Could you check a few things on this model? Use its own coordinates, in mm. A direction names the side the tool comes from. Give positions to 0.01 mm unless a question says otherwise; leave off trailing zeros. Order: outer loops, then holes, each group sorted by start corner. A loop starts at its lowest first (then second) coordinate and runs counter-clockwise, first axis right, second up. Notation, with made-up numbers: M 1,-39.5 L 24,-39.5 A23 cw 24,-8.5 Z; hole C 46.25,-0.75 d6. An arc over 180 degrees is marked long. Answer in a Markdown table with one row per item. Add a question column.
Autodesk Inventor part; units mm, degrees
ref_plane "YZ Plane" through (0, 0, 0) normal (1, 0, 0) x (0, 1, 0)
ref_plane "XZ Plane" through (0, 0, 0) normal (0, 1, 0) x (-1, 0, 0)
ref_plane "XY Plane" through (0, 0, 0) normal (0, 0, 1) x (1, 0, 0)
sketch "スケッチ1" plane through (0, 0, 0) normal (0, 1, 0) x (-1, 0, 0)
  circle A0 centre (15, 44.75) radius 2
  circle A1 centre (5, 44.75) radius 2
  circle A2 centre (10, 30) radius 3
  circle A3 centre (15, -4.75) radius 2
  circle A4 centre (5, -4.75) radius 2
  circle A5 centre (10, 30) radius 3
  line L0 (0, 0) -> (0, 40)
  line L1 (20, 0) -> (0, 0)
  line L2 (20, 40) -> (20, 0)
  line L3 (0, 40) -> (20, 40)
  line L4 (0, 40) -> (20, 40)
  line L5 (20, 45.25) -> (20, 40)
  arc A6 (20, 45.25) -> (18, 47.447) centre (18.0097, 45.4471) ccw
  line L6 (2, 47.447) -> (18, 47.447)
  arc A7 (2, 47.447) -> (0, 45.25) centre (1.9903, 45.4471) ccw
  line L7 (0, 40) -> (0, 45.25)
  circle A8 centre (15, 44.75) radius 2
  circle A9 centre (5, 44.75) radius 2
  line L8 (20, 0) -> (0, 0)
  line L9 (0, -5.25) -> (0, 0)
  arc A10 (0, -5.25) -> (2, -7.25) centre (2, -5.25) ccw
  line L10 (18, -7.25) -> (2, -7.25)
  arc A11 (18, -7.25) -> (20, -5.25) centre (18, -5.25) ccw
  line L11 (20, 0) -> (20, -5.25)
  circle A12 centre (5, -4.75) radius 2
  circle A13 centre (15, -4.75) radius 2
  line L12 (-8, 50.197) -> (28, 50.197)
  line L13 (30, 48.197) -> (30, -7.803)
  line L14 (28, -9.803) -> (-8, -9.803)
  line L15 (-10, -7.803) -> (-10, 48.197)
  arc A14 (30, 48.197) -> (28, 50.197) centre (28, 48.197) ccw
  arc A15 (-8, 50.197) -> (-10, 48.197) centre (-8, 48.197) ccw
  arc A16 (-10, -7.803) -> (-8, -9.803) centre (-8, -7.803) ccw
  arc A17 (28, -9.803) -> (30, -7.803) centre (28, -7.803) ccw
  line L16 (45.2724, 20.197) -> (-29.952, 20.197)
  line L17 (25, 53.3822) -> (25, -21.2286)
  line L18 (-5, 50.197) -> (-5, -9.803)
  line L19 (6.5, 45) -> (13.5, 45)
  line L20 (13.5, 45) -> (13.5, 40)
  line L21 (6.5, 40) -> (6.5, 45)
  line L22 (0, 40) -> (20, 40)
  point P0 (0, -4.75)
  point P1 (-10, 50.197)
  point P2 (30, -9.803)
  point P3 (30, 50.197)
  point P4 (10, 47.447)
  point P5 (10, 50.197)
  point P6 (-5, 20.197)
  point P7 (-5, 20.197)
  point P8 (25, 20.197)
  point P9 (25, 50.197)
  point P10 (25, -9.803)
  dimension "d0" = 40
  dimension "d1" = 60
  dimension "d2" = 2.75
  dimension "d3" = 10
  dimension "d4" = 2
  dimension "d5" = 30
  dimension "d6" = 5
  dimension "d7" = 5
  dimension "d8" = 60
  dimension "d9" = 0
  dimension "d22" = 2.75
  dimension "d23" = 2
  dimension "d24" = 2
  dimension "d25" = 10
  dimension "d26" = 15
  dimension "d27" = 5.447
  dimension "d28" = 10
  dimension "d29" = 20
  dimension "d30" = 20.197
extrude "押し出し1" add sketch "スケッチ1" along normal blind 5 contours A0 L20 L19 | A0 L19 A1 L21 L3 L7 A7 L6 A6 L5 L20 | L19 L21 A1 | L5 A6 L6 A7 L7 L0 L16 L18 L12 L17 L2 | L16 L17 L14 L18 L0 L9 A10 L10 A11 L11 L2 | L11 A11 L10 A10 L9 L1 | L17 L12 A14 L13 L16 | L16 L13 A17 L14 L17 | L18 L14 A16 L15 L16 | L16 L15 A15 L12 L18 | A3 | A4 picked at (15.8139, 44.6736) picked at (4.1802, 44.7383)
hole "穴1" at (5, 0, 20.197) at (-25, 0, 20.197) direction (0, 1, 0) diameter 4 end through all
sketch "スケッチ2" plane through (0, 5, 0) normal (0, 1, 0) x (1, 0, 0)
  circle A0 centre (5, -20.197) radius 2
  circle A1 centre (-25, -20.197) radius 2
  line L0 (-28, -50.197) -> (8, -50.197)
  arc A2 (8, -50.197) -> (10, -48.197) centre (8, -48.197) ccw
  line L1 (10, -48.197) -> (10, 7.803)
  arc A3 (10, 7.803) -> (8, 9.803) centre (8, 7.803) ccw
  line L2 (8, 9.803) -> (-28, 9.803)
  arc A4 (-28, 9.803) -> (-30, 7.803) centre (-28, 7.803) ccw
  line L3 (-30, 7.803) -> (-30, -48.197)
  arc A5 (-30, -48.197) -> (-28, -50.197) centre (-28, -48.197) ccw
  line L4 (-20, -40) -> (-20, 0)
  line L5 (-20, 0) -> (0, 0)
  line L6 (0, 0) -> (0, -40)
  line L7 (0, -40) -> (-6.5, -40)
  line L8 (-6.5, -40) -> (-6.5, -45)
  line L9 (-6.5, -45) -> (-13.5, -45)
  line L10 (-13.5, -45) -> (-13.5, -40)
  line L11 (-13.5, -40) -> (-20, -40)
  line L12 (-6, -40.5) -> (0.5, -40.5)
  line L13 (0.5, -40.5) -> (0.5, 0.5)
  line L14 (0.5, 0.5) -> (-20.5, 0.5)
  line L15 (-20.5, 0.5) -> (-20.5, -40.5)
  line L16 (-20.5, -40.5) -> (-14, -40.5)
  line L17 (-14, -40.5) -> (-14, -45.5)
  line L18 (-14, -45.5) -> (-6, -45.5)
  line L19 (-6, -45.5) -> (-6, -40.5)
  dimension "d19" = 0.5
extrude "押し出し2" cut sketch "スケッチ2" against normal blind 10 contours L19 L18 L17 L16 L15 L14 L13 L12
sketch "スケッチ3" plane through (0, 5, 0) normal (0, 1, 0) x (1, 0, 0)
  line L0 (10, -48.197) -> (10, 7.803)
  arc A0 (8, -50.197) -> (10, -48.197) centre (8, -48.197) ccw
  line L1 (-28, -50.197) -> (8, -50.197)
  arc A1 (-30, -48.197) -> (-28, -50.197) centre (-28, -48.197) ccw
  line L2 (-30, 7.803) -> (-30, -48.197)
  arc A2 (-28, 9.803) -> (-30, 7.803) centre (-28, 7.803) ccw
  line L3 (8, 9.803) -> (-28, 9.803)
  arc A3 (10, 7.803) -> (8, 9.803) centre (8, 7.803) ccw
  line L4 (6.2, -46.397) -> (6.2, 6.003)
  line L5 (6.2, 6.003) -> (-26.2, 6.003)
  line L6 (-26.2, 6.003) -> (-26.2, -46.397)
  line L7 (-26.2, -46.397) -> (6.2, -46.397)
  point P0 (0, 0)
  dimension "d31" = 3.8
extrude "押し出し3" cut sketch "スケッチ3" against normal blind 3
equation "\"d5\" = 0.5 * d1"
equation "\"d6\" = 0.5 * d3"
equation "\"d8\" = d1"
properties part number "servo_cover2_3D プリント"
1. Suppose I cut it at A-A on y = 1.05. List the corners of the cut face in (x, z) for me.
2. Suppose I cut it at B-B on x = -25. List the corners of the cut face in (y, z) for me.
3. Thinking about a two-plate mould opening in X: for faces 1 (the flat face through (7.5, 2, 19.8)), 2 (the flat face through (-26.2, 4, 34)), 3 (the flat face through (-10, 3, 45.5)), 4 (the cylindrical face through (9.43, 0.986, 49.596)), which applies, pulls with the +X half, pulls with the -X half, needs draft (parallel to the pull), parting line crosses it, or undercut?
4. Suppose I cut it at C-C on z = 6. List the corners of the cut face in (x, y) for me, plus the area to 3 significant figures.
5. Suppose I cut it at D-D on y = 4.3. List the corners of the cut face in (x, z) for me.
6. If I drill on line 1 along Z through (x, y) = (-13.5, 0.85); line 2 along Z through (x, y) = (-4, 4.25); line 3 along X through (y, z) = (1.15, 1), over which ranges is the centre line in solid material (lowest first)? Write a range as [from, to].
7. Will these pins go through, and if not, where does the flat tip stop? P1, Ø1.5, axis at y = 3.5, z = 42, coming from the +X side; P2, Ø1.5, axis at x = -6.5, y = 3, coming from the +Z side; P3, Ø0.9, axis at y = 3, z = 38, coming from the -X side; P4, Ø3, axis at x = -25, z = 20.197, coming from the +Y side.
8. For faces 5 (the flat face through (6.2, 4, 6)), 6 (the flat face through (-14, 3, 43)), 7 (the flat face through (-10, 4, 46.397)), 8 (the flat face through (-26.2, 4, 6)), which set-ups out of +Z, -Z, +X, -X, +Y, -Y let a thin tool reach every point of the face, with its end or its side?
Findings below:
| question | item | result |
|---|---|---|
| 1 | outline | M -30,-7.8 A2 ccw -28,-9.8 L 8,-9.8 A2 ccw 10,-7.8 L 10,48.2 A2 ccw 8,50.2 L -28,50.2 A2 ccw -30,48.2 Z; hole C -25,20.2 d4; hole M -20.5,-0.5 L 0.5,-0.5 L 0.5,40.5 L -6,40.5 L -6,45.5 L -14,45.5 L -14,40.5 L -20.5,40.5 Z; hole C 5,20.2 d4 |
| 2 | outline | M 0,-9.8 L 2,-9.8 L 2,-6 L 5,-6 L 5,18.2 L 0,18.2 Z; M 0,22.2 L 5,22.2 L 5,46.4 L 2,46.4 L 2,50.2 L 0,50.2 Z |
| 3 | face 1 | needs draft |
| 3 | face 2 | pulls with the -X half |
| 3 | face 3 | undercut |
| 3 | face 4 | pulls with the +X half |
| 4 | outline | M -30,0 L -20.5,0 L -20.5,5 L -26.2,5 L -26.2,2 L -30,2 Z; M 0.5,0 L 10,0 L 10,2 L 6.2,2 L 6.2,5 L 0.5,5 Z |
| 4 | area | 72.2 mm2 |
| 5 | outline | M -26.2,-6 L 6.2,-6 L 6.2,18.6 A2 cw long 6.2,21.8 L 6.2,46.4 L -26.2,46.4 L -26.2,21.8 A2 cw long -26.2,18.6 Z; hole M -20.5,-0.5 L 0.5,-0.5 L 0.5,40.5 L -6,40.5 L -6,45.5 L -14,45.5 L -14,40.5 L -20.5,40.5 Z |
| 6 | line 1 | [-9.8, -0.5], [45.5, 50.2] |
| 6 | line 2 | [-6, -0.5], [40.5, 46.4] |
| 6 | line 3 | [-30, -20.5], [0.5, 10] |
| 7 | P1 | x = 6.2 |
| 7 | P2 | z = 46.4 |
| 7 | P3 | x = -26.2 |
| 7 | P4 | through |
| 8 | face 5 | +Z, -Z, +X, +Y |
| 8 | face 6 | +Y, -Y |
| 8 | face 7 | +Z, +X, -X, +Y |
| 8 | face 8 | +Z, -Z, -X, +Y |
